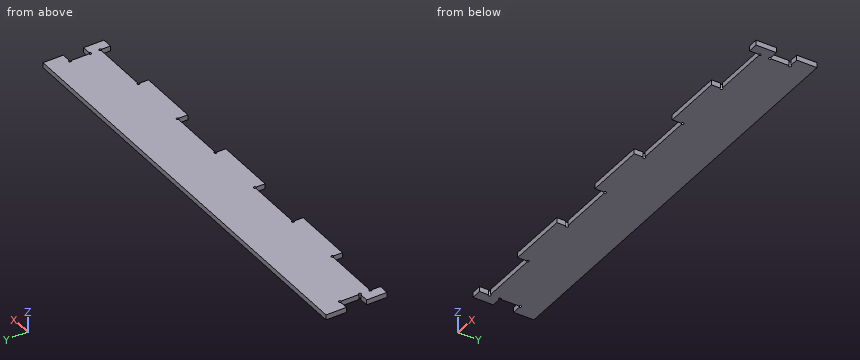
Autodesk Inventor part; units mm, degrees
ref_plane "YZ Plane" through (0, 0, 0) normal (1, 0, 0) x (0, 1, 0)
ref_plane "XZ Plane" through (0, 0, 0) normal (0, 1, 0) x (-1, 0, 0)
ref_plane "XY Plane" through (0, 0, 0) normal (0, 0, 1) x (1, 0, 0)
sketch "Sketch1" plane through (0, 0, 0) normal (0, 0, 1) x (1, 0, 0)
  line L0 (-173, 24) -> (173, 24)
  line L1 (173, 24) -> (173, -24)
  line L2 (173, -24) -> (-173, -24)
  line L3 (-173, -24) -> (-173, 24)
  point P0 (0, 0)
  point P1 (173, 0)
  point P2 (0, 24)
  dimension "d0" = 48
  dimension "d1" = 346
extrude "Extrusion1" add sketch "Sketch1" along normal blind 4
sketch "Esboço2" plane through (0, 0, 4) normal (0, 0, 1) x (1, 0, 0)
  line L0 (-165, -24) -> (-118.5, -24)
  line L1 (-118.5, -24) -> (-118.5, -16)
  line L2 (-118.5, -16) -> (-165, -16)
  line L3 (-165, -16) -> (-165, -24)
  line L4 (-173, 24) -> (-173, -24)
  line L5 (-70.5, -24) -> (-24, -24)
  line L6 (-24, -24) -> (-24, -16)
  line L7 (-24, -16) -> (-70.5, -16)
  line L8 (-70.5, -16) -> (-70.5, -24)
  circle A0 centre (-24, -16) radius 1
  circle A1 centre (-70.5, -16) radius 1
  circle A2 centre (-118.5, -16) radius 1
  circle A3 centre (-165, -16) radius 1
  line L9 (-173, -24) -> (173, -24)
  point P0 (0, 0)
  dimension "d4" = 46.5
  dimension "d7" = 46.5
  dimension "d8" = 48
  dimension "d14" = 2
  dimension "d15" = 2
  dimension "d16" = 2
  dimension "d20" = 8
  dimension "d21" = 8
  dimension "d22" = 0
extrude "Extrusão2" cut sketch "Esboço2" against normal blind 10
mirror "Espelhamento1" about plane through (0, 0, 0) normal (1, 0, 0) of "Extrusão2"
sketch "Esboço3" plane through (0, 0, 4) normal (0, 0, 1) x (1, 0, 0)
  line L0 (-173, 24) -> (-173, -24)
  line L1 (-173, -8) -> (-165, -8)
  line L2 (-165, -8) -> (-165, 8)
  line L3 (-165, 8) -> (-173, 8)
  line L4 (-173, 8) -> (-173, -8)
  line L5 (-173, -24) -> (-165, -24)
  line L6 (173, 24) -> (-173, 24)
  circle A0 centre (-165, 8) radius 1
  circle A1 centre (-165, -8) radius 1
  point P0 (0, 0)
  dimension "d23" = 8
  dimension "d24" = 16
  dimension "d25" = 16
  dimension "d26" = 16
  dimension "d27" = 2
  dimension "d28" = 2
extrude "Extrusão3" cut sketch "Esboço3" against normal blind 10
mirror "Espelhamento2" about plane through (0, 0, 0) normal (1, 0, 0) of "Extrusão3"
properties part number "frente inferior"
Can you work these out from the model? Positions are in its coordinate system, mm. Coordinates: 2 decimals unless noted, no trailing zeros. Write each loop counter-clockwise with the first axis right and the second up, starting at its lowest first coordinate (ties: lowest second). Pieces come first, ordered by that corner, then holes. Notation, with made-up numbers: (13.25, 65.5) -> (64.25, 65.5) arc R21 ccw to (64.25, 81.5) -> close; hole circle Ø6 at (55.5, -32). An arc over 180 degrees is marked (long way). Write item = value, one per line.
(1) Imagine slicing it at B-B (x = 50.5). Please give me the cut outline in (y, z).
Verdict:
outline = (-16, 0) -> (24, 0) -> (24, 4) -> (-16, 4) -> close
(2) For pin 1 (12 mm diameter, centred on x = -81, y = 10.5, fed in from -Z); pin 2 (1.2 mm diameter, centred on y = -2.5, z = 1.5, fed in from -X); pin 3 (1.8 mm diameter, centred on x = 24, y = -16, fed in from -Z); pin 4 (1.5 mm diameter, centred on x = -60, z = 1.5, fed in from -Y), each with a flat end and sliding along its axis, tell me the tip position at first contact or that it passes through.
Verdict:
pin_1 = 0
pin_2 = -165
pin_3 = through
pin_4 = -16
(3) Imagine slicing it at A-A (y = 1). Please give me the cut outline in (x, z), and give its area (3 significant figures).
Verdict:
outline = (-165, 0) -> (165, 0) -> (165, 4) -> (-165, 4) -> close
area = 1,320 mm^2
(4) If I drill on probe 1 along X at (y, z) = (-20, 0.9); probe 2 along X at (y, z) = (5.5, 1.7); probe 3 along Y at (x, z) = (147, 0.7), over which ranges is the centre line in solid material (lowest first)?
Verdict:
probe_1 = -173 to -165, -118.5 to -70.5, -24 to 24, 70.5 to 118.5, 165 to 173
probe_2 = -165 to 165
probe_3 = -16 to 24
